Can you work these out from the model? Positions are in its coordinate system, mm. Give positions to 0.01 mm unless a question says otherwise; leave off trailing zeros. Write each loop counter-clockwise with the first axis right and the second up, starting at its lowest first coordinate (ties: lowest second). Pieces come first, ordered by that corner, then holes. Notation, with made-up numbers: M 63,73 L 73,73 A22 cw 73,97 Z; hole C 14.5,41 d5. An arc over 180 degrees is marked long. Use CSV: the item, a comma, the result in double quotes. Start each with the question number.
from build123d import *

# Parameters (mm, degrees)
SKETCH1_W           = 95
SKETCH1_H           = 135
BOSS_EXTRUDE1_DEPTH = 5
SKETCH3_W           = 80
SKETCH3_H           = 120
CUT_EXTRUDE1_DEPTH  = 99.930888994
SKETCH4_W           = 7
SKETCH4_H           = 6
BOSS_EXTRUDE4_DEPTH = 2.5
SKETCH6_W           = 7.5
SKETCH6_H           = 7.8
BOSS_EXTRUDE5_DEPTH = 5
SKETCH7_R           = 1.95
CUT_EXTRUDE2_DEPTH  = 10
SKETCH16_W          = 7.5
SKETCH16_H          = 15
BOSS_EXTRUDE9_DEPTH = 12
SKETCH18_W          = 12
SKETCH18_H          = 10
CUT_EXTRUDE3_DEPTH  = 1002


with BuildPart() as part:
    # Sketch1 → Boss-Extrude1 (new body)
    with BuildSketch(Plane(origin=(0, 0, 0), x_dir=(1, 0, 0), z_dir=(0, 1, 0))):
        with Locations((-15.327225131, -8.756544503)):
            Rectangle(SKETCH1_W, SKETCH1_H)
    extrude(amount=BOSS_EXTRUDE1_DEPTH)

    # Sketch3 → Cut-Extrude1 (cut, through all)
    with BuildSketch(Plane(origin=(0, 5, 0), x_dir=(1, 0, 0), z_dir=(0, 1, 0))):
        with Locations((-15.327225131, -8.756544503)):
            Rectangle(SKETCH3_W, SKETCH3_H)
    extrude(amount=-CUT_EXTRUDE1_DEPTH, mode=Mode.SUBTRACT)

    # Sketch4 → Boss-Extrude4 (add)
    with BuildSketch(Plane(origin=(0, 5, 0), x_dir=(1, 0, 0), z_dir=(0, 1, 0))):
        with Locations((-51.827225131, 48.243455497)):
            Rectangle(SKETCH4_W, SKETCH4_H)
        with Locations((21.172774869, -65.756544503)):
            Rectangle(SKETCH4_W, SKETCH4_H)
        with Locations((21.172774869, 48.243455497)):
            Rectangle(SKETCH4_W, SKETCH4_H)
        with Locations((-51.827225131, -65.756544503)):
            Rectangle(SKETCH4_W, SKETCH4_H)
        with Locations((-51.827225131, -8.756544503)):
            Rectangle(SKETCH4_W, SKETCH4_H)
        with Locations((21.172774869, -8.756544503)):
            Rectangle(SKETCH4_W, SKETCH4_H)
    extrude(amount=-BOSS_EXTRUDE4_DEPTH)

    # Sketch6 → Boss-Extrude5 (add)
    with BuildSketch(Plane.XZ):
        with Locations((28.422774869, -62.643455497)):
            Rectangle(SKETCH6_W, SKETCH6_H)
        with Locations((-59.077225131, -62.643455497)):
            Rectangle(SKETCH6_W, SKETCH6_H)
    extrude(amount=-BOSS_EXTRUDE5_DEPTH)

    # Sketch7 → Cut-Extrude2 (cut)
    with BuildSketch(Plane(origin=(0, 0, 0), x_dir=(-1, 0, 0), z_dir=(0, -1, 0))):
        with Locations(Location((59.077225131, 62.643455497, 0), (0, 0, 90))):
            Circle(SKETCH7_R)
        with Locations(Location((-28.422774869, 62.643455497, 0), (0, 0, 90))):
            Circle(SKETCH7_R)
    extrude(amount=-CUT_EXTRUDE2_DEPTH, mode=Mode.SUBTRACT)

    # Sketch16 → Boss-Extrude9 (add)
    with BuildSketch(Plane(origin=(0, 0, 0), x_dir=(-1, 0, 0), z_dir=(0, -1, 0))):
        with Locations((59.077225131, -43.756544503)):
            Rectangle(SKETCH16_W, SKETCH16_H)
        with Locations((-28.422774869, -43.756544503)):
            Rectangle(SKETCH16_W, SKETCH16_H)
    extrude(amount=BOSS_EXTRUDE9_DEPTH)

    # Sketch18 → Cut-Extrude3 (cut)
    with BuildSketch(Plane.ZY.offset(62.827225131)):
        with Locations((43.756544503, -6)):
            Rectangle(SKETCH18_W, SKETCH18_H)
    extrude(amount=-CUT_EXTRUDE3_DEPTH, mode=Mode.SUBTRACT)


solid = part.part
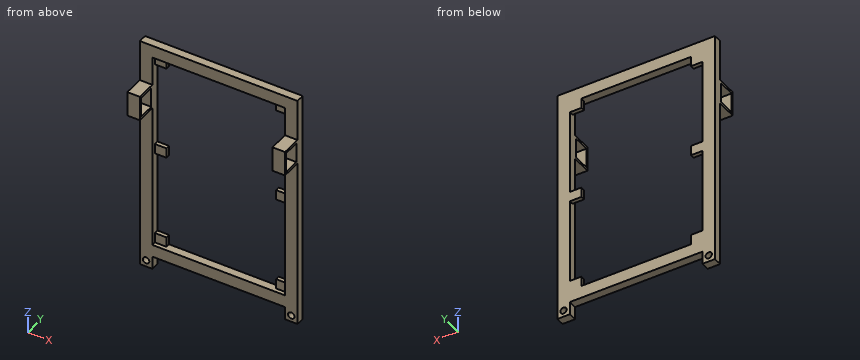
(1) Will these pins go through, and if not, where does the flat tip stop? pin 1 Ø2.5 at (x, y) = (-7, 3.5) entering from -Z; pin 2 Ø6 at (x, y) = (-58, -3.5) entering from -Z; pin 3 Ø5 at (x, z) = (20.5, 66.5) entering from -Y.
(2) I want a section at A-A (z = 47). Write out the boundary of the cut face in (x, y), and give its area (3 significant figures).
(3) I want a section at B-B (x = 13). Write out the boundary of the cut face in (y, z).
(4) I want a section at C-C (z = 31). Write out the boundary of the cut face in (x, y).
(5) I want a section at D-D (y = -3). Write out the boundary of the cut face in (x, z).
(6) Please list where these lines run through material, in increasing order: L1, parallel to X at y = 3, z = 48; L2, parallel to Z at x = -23, y = 2; L3, parallel to Y at x = 20, z = -48.5. Write a range as [from, to].
Geometry results:
1,pin 1,"stops at z = -58.74"
1,pin 2,"stops at z = 36.26"
1,pin 3,"stops at y = 0"
2,outline,"M -62.83,-12 L -55.33,-12 L -55.33,-11 L -62.83,-11 Z; M -62.83,-1 L -55.33,-1 L -55.33,5 L -62.83,5 Z; M 24.67,-12 L 32.17,-12 L 32.17,-11 L 24.67,-11 Z; M 24.67,-1 L 32.17,-1 L 32.17,5 L 24.67,5 Z"
2,area,"105 mm2"
3,outline,"M 0,-58.74 L 5,-58.74 L 5,-51.24 L 0,-51.24 Z; M 0,68.76 L 5,68.76 L 5,76.26 L 0,76.26 Z"
4,outline,"M -62.83,0 L -55.33,0 L -55.33,5 L -62.83,5 Z; M 24.67,0 L 32.17,0 L 32.17,5 L 24.67,5 Z"
5,outline,"M -62.83,36.26 L -55.33,36.26 L -55.33,37.76 L -62.83,37.76 Z; M -62.83,49.76 L -55.33,49.76 L -55.33,51.26 L -62.83,51.26 Z; M 24.67,36.26 L 32.17,36.26 L 32.17,37.76 L 24.67,37.76 Z; M 24.67,49.76 L 32.17,49.76 L 32.17,51.26 L 24.67,51.26 Z"
6,L1,"x = [-62.83, -55.33], [24.67, 32.17]"
6,L2,"z = [-58.74, -51.24], [68.76, 76.26]"
6,L3,"y = [2.5, 5]"
